Geometry: final body of the model. Coordinates: model frame, mm. A direction names the side the tool comes from. Round coordinates to 2 decimals unless told otherwise and drop trailing zeros. Loops run counter-clockwise (first coordinate to the right, second up) from the corner with the lowest first, then second, coordinate; pieces in that order, holes last. Notation, with made-up numbers: M 84,-2.5 L 125,-2.5 A15 cw 125,12.5 Z; hole C 40.5,28.5 d3. An arc over 180 degrees is marked long. Answer as a JSON object with one key per item and string values.
from build123d import *

# Parameters (mm, degrees)
EXTRUDE_1_DEPTH = 96
EXTRUDE_2_DEPTH = 8


with BuildPart() as part:
    # Эскиз1 → Бобышка-Вытянуть1 (new body)
    with BuildSketch(Plane(origin=(0, 0, 0), x_dir=(0, 0, -1), z_dir=(1, 0, 0))):
        Polygon((0, 109.262066559), (60, 37.756851003), (60, -25.242859431), (50, -25.242859431), (50, 24.757140569), (10, 24.757140569), (10, -25.242859431), (0, -25.242859431), align=None)
    extrude(amount=EXTRUDE_1_DEPTH)

    # Эскиз3 → Бобышка-Вытянуть2 (add)
    with BuildSketch(Plane(origin=(0, 45.144453906, -53.801065128), x_dir=(-1, 0, 0), z_dir=(0, 0.6427876096865404, -0.7660444431189771))):
        Polygon((-96, -1.355361582), (-96, -9.643830681), (0, -9.643830681), (0, -1.355361582), (-3, -1.355361582), (-3, -6.643830681), (-93, -6.643830681), (-93, -1.355361582), align=None)
    extrude(amount=EXTRUDE_2_DEPTH)


solid = part.part
1) Section query C-C (z = -8.5). Return the cut outline in (x, y), and give its area (3 significant figures).
Results:
{"outline": "M 0,-25.24 L 96,-25.24 L 96,99.13 L 0,99.13 Z", "area": "11,900 mm2"}
2) Ray query, line 1 (Z direction, x = 13, y = 23.5); line 2 (Z direction, x = 34.5, y = 29.5); line 3 (Z direction, x = 50, y = 94.5). Return the intervals inside material, ascending.
Results:
{"line 1": "-60 to -50, -10 to 0", "line 2": "-60 to 0", "line 3": "-12.39 to 0"}
3) Section query A-A (y = 3). Return the cut outline in (x, z), and give its area (3 significant figures).
Results:
{"outline": "M 0,-60 L 96,-60 L 96,-50 L 0,-50 Z; M 0,-10 L 96,-10 L 96,0 L 0,0 Z", "area": "1,920 mm2"}
4) Section query D-D (y = 85). Return the cut outline in (x, z).
Results:
{"outline": "M 0,-20.36 L 96,-20.36 L 96,0 L 0,0 Z"}
5) Pin query (flat end, axial travel): P1, Ø3, axis at x = 46, y = 77.5, coming from the +Z side; P2, Ø1, axis at x = 22.5, z = -43.5, coming from the -Y side; P3, Ø2, axis at x = 18.5, z = -32.5, coming from the +Y side. Return the tip coordinate at first contact, or that it passes through.
Results:
{"P1": "z = 0", "P2": "y = 24.76", "P3": "y = 71.72"}
6) Section query B-B (x = 37). Return the cut outline in (y, z), and give its area (3 significant figures).
Results:
{"outline": "M -25.24,-60 L 37.76,-60 L 42.9,-66.13 L 45.2,-64.2 L 40.05,-58.07 L 109.26,0 L -25.24,0 L -25.24,-10 L 24.76,-10 L 24.76,-50 L -25.24,-50 Z", "area": "3,950 mm2"}
7) Pull-direction query (Z, two-part tool) for faces 1 (the flat face through (47, 7, -60)), 2 (the flat face through (0, 36, -24)), 3 (the flat face through (47, -1, -50)); classes: +Z half, -Z half, draft (parallel to the pull), parting line (faces both ways), or undercut.
Results:
{"face 1": "-Z half", "face 2": "draft", "face 3": "undercut"}
8) Reachability of faces 4 (the flat face through (3, 45, -59)), 5 (the flat face through (1.48, 46.64, -57.69)), 6 (the flat face through (47, 24.757, -30)), 7 (the flat face through (48.67, 40.29, -63.02)) from +Z, -Z, +X, -X, +Y, -Y: full face, straight path, thin tool, end or side. Return the list, or none.
Results:
{"face 4": "+Y", "face 5": "+X, -X, +Y", "face 6": "+X, -X, -Y", "face 7": "-Z, +X, -X, -Y"}
